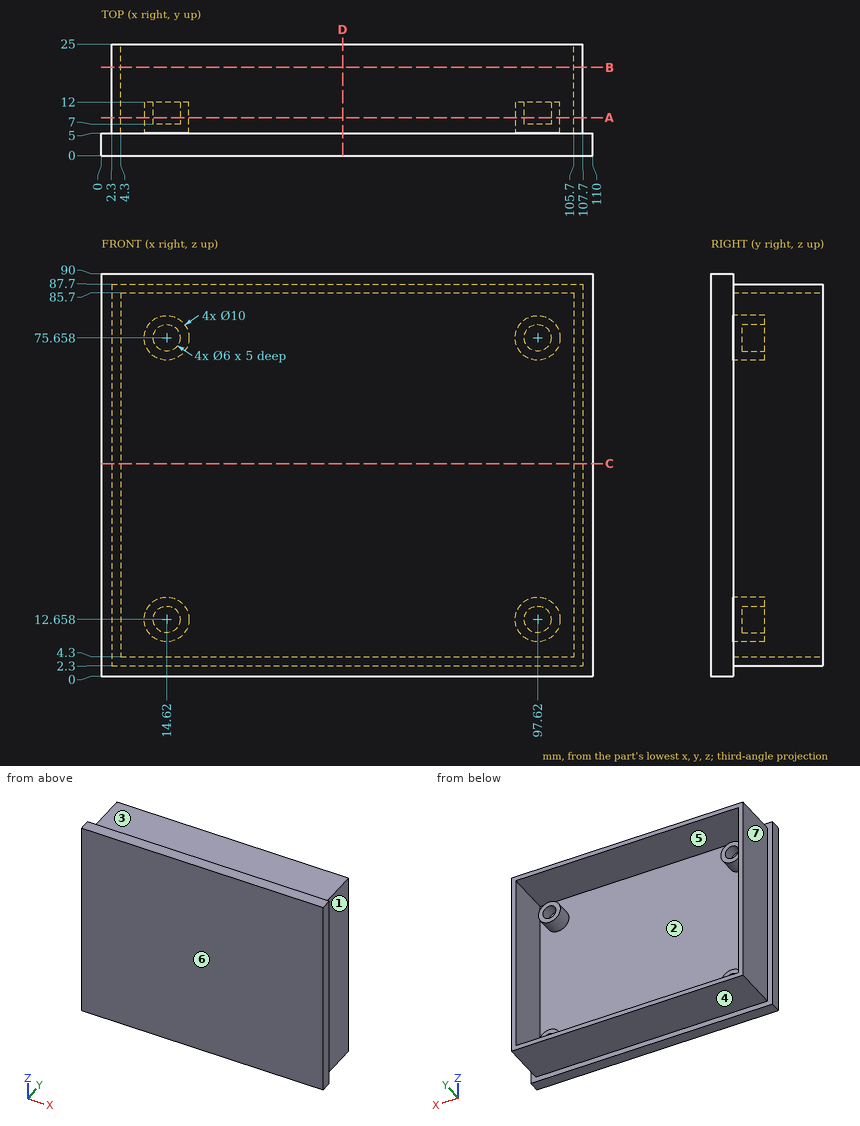
Input: dimensioned drawing with shaded views. Units: mm. Origin: part minimum x, y, z. A direction names the side the tool comes from. Give positions to 0.01 mm unless a question says otherwise; leave off trailing zeros. Loops run counter-clockwise (first coordinate to the right, second up) from the corner with the lowest first, then second, coordinate; pieces in that order, holes last. Notation, with made-up numbers: M 80,65.5 L 104,65.5 A24 cw 104,96.5 Z; hole C 3,40.25 d1. An arc over 180 degrees is marked long. Put each result on its own line as item: value. Start each with the question number.
1) Contact query for flat-ended pins moving along their axis: pin 1 (10 mm diameter, centred on x = 86, z = 27.5, fed in from +Y); pin 2 (3 mm diameter, centred on x = 98.5, z = 14, fed in from +Y); pin 3 (5 mm diameter, centred on x = 97.5, z = 13, fed in from +Y). Output: stop coordinate, or through.
2) Ray query, line 1 along X through (y, z) = (17.75, 76); line 2 along Z through (x, y) = (50, 7.75); line 3 along Y through (x, z) = (87, 22.5). Return the intervals inside material, ascending.
3) Cut plane C-C (z = 47.5). Output: boundary loops of the cut face in (x, y), then the cut area to 3 significant figures.
4) Cut plane D-D (x = 54). Output: boundary loops of the cut face in (y, z), then the cut area to 3 significant figures.
5) Cut plane B-B (y = 19.75). Output: boundary loops of the cut face in (x, z).
6) Cut plane A-A (y = 8.5). Give the number of separate pieces and of enclosed holes in the cut face.
7) Pull-direction query (Z, two-part tool) for the marked faces 1, 2 and 3; classes: pulls with the +Z half, pulls with the -Z half, needs draft (parallel to the pull), parting line crosses it, or undercut.
8) Access query for the marked faces 4, 5, 6 and 7. Directions: +Z, -Z, +X, -X, +Y, -Y. A direction counts if a zero-diameter tool reaches every point of the face in a straight line with its end or side. Return the directions, or none.
Verdict:
1. pin 1: y = 5
1. pin 2: y = 12
1. pin 3: y = 7
2. line 1: 2.3 to 4.3, 105.7 to 107.7
2. line 2: 2.3 to 4.3, 85.7 to 87.7
2. line 3: 0 to 5
3. outline: M 0,0 L 110,0 L 110,5 L 107.7,5 L 107.7,25 L 105.7,25 L 105.7,5 L 4.3,5 L 4.3,25 L 2.3,25 L 2.3,5 L 0,5 Z
3. area: 630 mm2
4. outline: M 0,0 L 5,0 L 5,2.3 L 25,2.3 L 25,4.3 L 5,4.3 L 5,85.7 L 25,85.7 L 25,87.7 L 5,87.7 L 5,90 L 0,90 Z
4. area: 530 mm2
5. outline: M 2.3,2.3 L 107.7,2.3 L 107.7,87.7 L 2.3,87.7 Z; hole M 4.3,4.3 L 105.7,4.3 L 105.7,85.7 L 4.3,85.7 Z
6. separate pieces: 5
6. enclosed holes: 5
7. face 1: needs draft
7. face 2: undercut
7. face 3: pulls with the +Z half
8. face 4: -Z, +X, -X, +Y
8. face 5: +Y
8. face 6: +Z, -Z, +X, -X, -Y
8. face 7: +Z, -Z, -X, +Y
